Design review of the part shown in the three views and the two pictorial views. Dimensions are in mm from the part's minimum x, y and z. Round coordinates to 2 decimals unless told otherwise and drop trailing zeros. Order: outer loops, then holes, each group sorted by start corner. A loop starts at its lowest first (then second) coordinate and runs counter-clockwise, first axis right, second up.
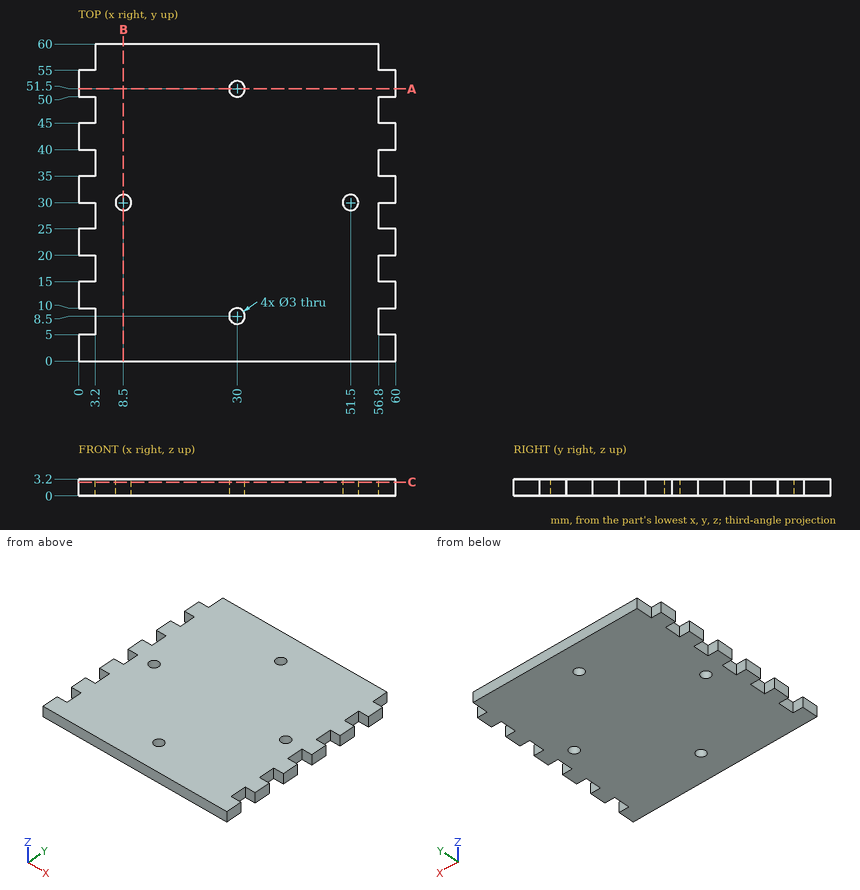
1) Take a section at C-C on z = 2.6. State how many separate pieces and enclosed holes the cut face has, plus the area to 3 significant figures.
Results:
separate pieces: 1
enclosed holes: 4
area: 3,380 mm2
2) Take a section at A-A on y = 51.5. Give the boundary of the cut face in (x, z), plus the area to 3 significant figures.
Results:
outline: (0, 0) - (28.5, 0) - (28.5, 3.2) - (0, 3.2) - close; (31.5, 0) - (60, 0) - (60, 3.2) - (31.5, 3.2) - close
area: 182 mm2
3) Clearance check with flat-ended pins moving along their axes: P1, Ø1, axis at y = 18, z = 1, coming from the +X side; P2, Ø1, axis at y = 27.5, z = 1, coming from the -X side; P3, Ø1, axis at x = 59, z = 2, coming from the +Y side. State where each tip first meets the part, or that it passes through.
Results:
P1: stops at x = 56.8
P2: stops at x = 3.2
P3: stops at y = 55
4) To check wall thickness, follow line 1 along Y through (x, z) = (30, 2.3); line 2 along Y through (x, z) = (8.5, 2.15); line 3 along X through (y, z) = (38, 2.2). State the ranges of each line that lie inside material, in increasing order.
Results:
line 1: y = 0 to 7, 10 to 50, 53 to 60
line 2: y = 0 to 28.5, 31.5 to 60
line 3: x = 3.2 to 56.8
